The model under review builds one solid part; all positions refer to its coordinate system, in mm. Face numbers are marked on the shaded views. A direction names the side the tool comes from. Give positions to 0.01 mm unless a question says otherwise; leave off trailing zeros. Order: outer loops, then holes, each group sorted by start corner. A loop starts at its lowest first (then second) coordinate and runs counter-clockwise, first axis right, second up. Notation, with made-up numbers: (-27, -24.5) -> (8, -24.5) arc R24 cw to (8, -12.5) -> close; hole circle Ø4 at (51, 64.25). An arc over 180 degrees is marked (long way). Use one line per item in the form item = value.
Autodesk Inventor part; units mm, degrees
ref_plane "YZ Plane" through (0, 0, 0) normal (1, 0, 0) x (0, 1, 0)
ref_plane "XZ Plane" through (0, 0, 0) normal (0, 1, 0) x (-1, 0, 0)
ref_plane "XY Plane" through (0, 0, 0) normal (0, 0, 1) x (1, 0, 0)
sketch "Sketch1" plane through (0, 0, 0) normal (0, 0, 1) x (1, 0, 0)
  line L0 (0, 0) -> (0, 40)
  line L1 (0, 0) -> (40, 0)
  dimension "d0" = 40
  dimension "d1" = 40
contour flange "Contour Flange1" sketch "Sketch1" thickness 1.5 bend radius 1.5 width 268 along (0, 0, 1) mid plane yes both sides no wall seen from (0, 20, 0) lies toward (1, 0, 0) curves L0 L1
bend "Bend1"
corner "Corner1"
equation "\"d2\" = BendReliefWidth"
equation "\"d3\" = BendReliefDepth"
equation "\"d4\" = MinimumRemnant"
equation "\"d5\" = BendRadius"
equation "\"d7\" = BendRadius"
equation "\"d9\" = CornerReliefSize"
equation "\"d10\" = GapSize"
equation "\"d11\" = JacobiRadiusSize"
equation "\"BendRadius\" = Thickness"
equation "\"BendReliefWidth\" = Thickness"
equation "\"BendReliefDepth\" = 0.5 * Thickness"
equation "\"CornerReliefSize\" = 4 * Thickness"
equation "\"MinimumRemnant\" = 2 * Thickness"
equation "\"TransitionRadius\" = BendRadius"
equation "\"JacobiRadiusSize\" = BendRadius"
equation "\"GapSize\" = Thickness"
properties part number "L 40x40x268" material "Stainless Steel"
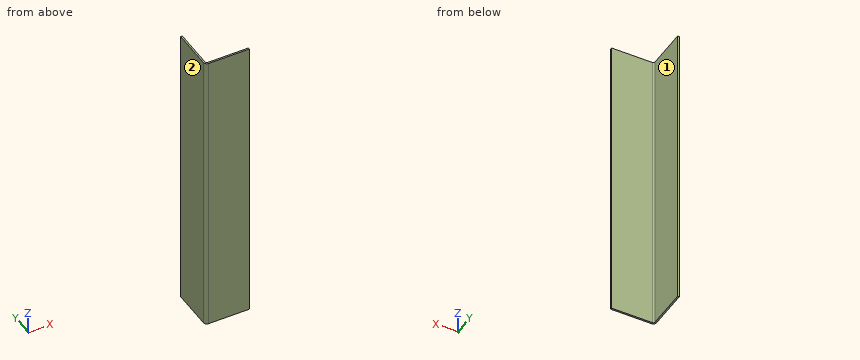
1. Add section A-A on z = -106. Give the boundary of the cut face in (x, y), then the cut area to 3 significant figures.
Values:
outline = (0, 3) arc R3 ccw to (3, 0) -> (40, 0) -> (40, 1.5) -> (3, 1.5) arc R1.5 cw to (1.5, 3) -> (1.5, 40) -> (0, 40) -> close
area = 116 mm^2
2. For pin 1 Ø2 at (x, z) = (7, -95) entering from +Y; pin 2 Ø2 at (y, z) = (32.5, 8.5) entering from +X, all flat-tipped, find the tip position at first contact; note any pin that passes through.
Values:
pin_1 = 1.5
pin_2 = 1.5
3. Add section B-B on x = 11. Give the boundary of the cut face in (y, z), then the cut area to 3 significant figures.
Values:
outline = (0, -134) -> (1.5, -134) -> (1.5, 134) -> (0, 134) -> close
area = 402 mm^2
4. For L1, parallel to X at y = 4, z = 89.5, list the stretches that pass through material, from the lowest coordinate up.
Values:
L1 = 0 to 1.5
5. Tool access review of the marked faces 1 and 2: name each direction out of +Z, -Z, +X, -X, +Y, -Y from which nothing blocks a thin tool from reaching the whole face with its end or side.
Values:
face_1 = +Z, -Z, +X, +Y
face_2 = +Z, -Z, -X, +Y, -Y
